Work out the finished part from the listing and answer in its coordinate system (mm). Round coordinates to 2 decimals unless told otherwise and drop trailing zeros. Write each loop counter-clockwise with the first axis right and the second up, starting at its lowest first coordinate (ties: lowest second). Pieces come first, ordered by that corner, then holes.
1. A flat-ended cylindrical pin translates along its axis: pin 1 Ø2.5 at (x, z) = (8.95, -5) entering from -Y. Find the tip coordinate at first contact, or state that the pin passes through.
2. Straight lines are drawn through the part: probe 1 along X at (y, z) = (3.25, 10); probe 2 along X at (y, z) = (6.5, -1); probe 3 along X at (y, z) = (4, 9). For each, find the intervals that lie inside material, in ascending order.
3. Find section D-D (z = -5). Write down the section's boundary in (x, y), and give its area (3 significant figures).
4. Find section A-A (x = 8.95). Write down the section's boundary in (y, z), and give its area (3 significant figures).
5. Find section B-B (y = 6.5). Write down the section's boundary in (x, z), and give its area (3 significant figures).
6. Find section C-C (z = -0.5). Write down the section's boundary in (x, y).
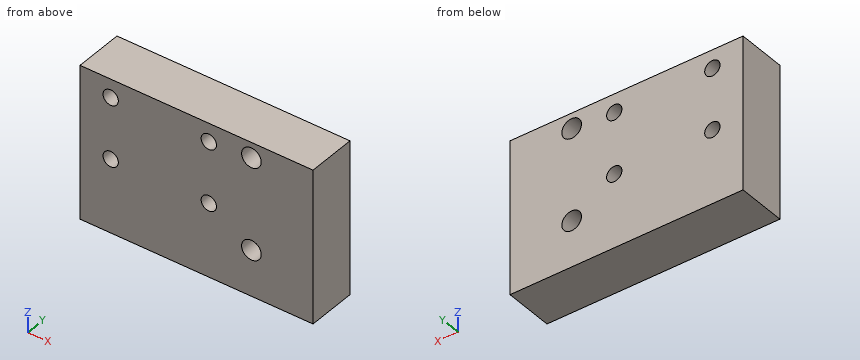
```python
from build123d import *

# Parameters (mm, degrees)
SKETCH_1_W          = 38
SKETCH_1_H          = 25
EXTRUDE_1_DEPTH     = 8
SKETCH_2_R          = 1.25
CUT_EXTRUDE_1_DEPTH = 25.109126902
SKETCH_4_R          = 1.6
CUT_EXTRUDE_2_DEPTH = 25.109126902


with BuildPart() as part:
    # 草图1 → 凸台-拉伸1 (new body)
    with BuildSketch(Plane(origin=(0, 0, 0), x_dir=(1, 0, 0), z_dir=(0, 1, 0))):
        Rectangle(SKETCH_1_W, SKETCH_1_H)
    extrude(amount=EXTRUDE_1_DEPTH)

    # 草图2 → 切除-拉伸1 (cut, through all)
    with BuildSketch(Plane.XZ):
        with Locations(Location((2, 9.5, 0), (0, 0, 270))):
            Circle(SKETCH_2_R)
        with Locations(Location((2, -0.5, 0), (0, 0, 270))):
            Circle(SKETCH_2_R)
        with Locations(Location((-14, 9.5, 0), (0, 0, 270))):
            Circle(SKETCH_2_R)
        with Locations(Location((-14, -0.5, 0), (0, 0, 270))):
            Circle(SKETCH_2_R)
    extrude(amount=-CUT_EXTRUDE_1_DEPTH, mode=Mode.SUBTRACT)

    # 草图4 → 切除-拉伸2 (cut, through all)
    with BuildSketch(Plane.XZ):
        with Locations(Location((8.95, 10, 0), (0, 0, 270))):
            Circle(SKETCH_4_R)
        with Locations(Location((8.95, -5, 0), (0, 0, 270))):
            Circle(SKETCH_4_R)
    extrude(amount=-CUT_EXTRUDE_2_DEPTH, mode=Mode.SUBTRACT)


solid = part.part
```
Worked answers:
1. pin 1: passes through
2. probe 1: x = -19 to -15.15, -12.85 to 0.85, 3.15 to 7.35, 10.55 to 19
2. probe 2: x = -19 to -15.15, -12.85 to 0.85, 3.15 to 19
2. probe 3: x = -19 to -15.15, -12.85 to 0.85, 3.15 to 7.7, 10.2 to 19
3. outline: (-19, 0) - (7.35, 0) - (7.35, 8) - (-19, 8) - close; (10.55, 0) - (19, 0) - (19, 8) - (10.55, 8) - close
3. area: 278 mm2
4. outline: (0, -12.5) - (8, -12.5) - (8, -6.6) - (0, -6.6) - close; (0, -3.4) - (8, -3.4) - (8, 8.4) - (0, 8.4) - close; (0, 11.6) - (8, 11.6) - (8, 12.5) - (0, 12.5) - close
4. area: 149 mm2
5. outline: (-19, -12.5) - (19, -12.5) - (19, 12.5) - (-19, 12.5) - close; hole circle Ø2.5 at (-14, -0.5); hole circle Ø2.5 at (-14, 9.5); hole circle Ø2.5 at (2, -0.5); hole circle Ø2.5 at (2, 9.5); hole circle Ø3.2 at (8.95, -5); hole circle Ø3.2 at (8.95, 10)
5. area: 914 mm2
6. outline: (-19, 0) - (-15.25, 0) - (-15.25, 8) - (-19, 8) - close; (-12.75, 0) - (0.75, 0) - (0.75, 8) - (-12.75, 8) - close; (3.25, 0) - (19, 0) - (19, 8) - (3.25, 8) - close
